Source: CAD feature listing. Evaluate the final solid. Frame: model axes, mm. A direction names the side the tool comes from. Round coordinates to 2 decimals unless told otherwise and drop trailing zeros. Write each loop counter-clockwise with the first axis right and the second up, starting at its lowest first coordinate (ties: lowest second). Pieces come first, ordered by that corner, then holes. Notation, with made-up numbers: (75.25, 22) -> (119.25, 22) arc R14 cw to (119.25, 26) -> close; hole circle Ø6 at (-28.5, -17). An arc over 180 degrees is marked (long way). Put each result on its own line as item: value.
```python
from build123d import *

# Parameters (mm, degrees)
SKETCH2_R           = 0.875
BOSS_EXTRUDE1_DEPTH = 1


with BuildPart() as part:
    # Sketch2 → Boss-Extrude1 (new body)
    with BuildSketch(Plane.XY):
        with BuildLine():
            Line((-5.603408365, 96.42556159), (-5.603408365, 30.425568858))
            ThreePointArc((-5.603408365, 30.425568858), (-4.43183549, 27.597141733), (-1.603408365, 26.425568858))
            Line((-1.603408365, 26.425568858), (41.250894393, 26.425568858))
            ThreePointArc((41.250894393, 26.425568858), (52.580802046, 23.710837368), (61.450097132, 16.156224264))
            Line((61.450097132, 16.156224264), (63.436905361, 13.431841599))
            ThreePointArc((63.436905361, 13.431841599), (64.629324911, 12.347724535), (66.15279536, 11.822165805))
            Line((66.15279536, 11.822165805), (84.159730921, 9.479779923))
            ThreePointArc((84.159730921, 9.479779923), (103.351530482, 5.02611066), (121.297670701, -3.103858071))
            Line((121.297670701, -3.103858071), (122.126093986, -3.582626958))
            ThreePointArc((122.126093986, -3.582626958), (125.162033535, -3.98331921), (127.591695632, -2.119391819))
            Line((127.591695632, -2.119391819), (143.453487011, 25.354036748))
            ThreePointArc((143.453487011, 25.354036748), (143.853088701, 26.318760568), (143.989385396, 27.354036748))
            Line((143.989385396, 27.354036748), (143.989385396, 98.790469349))
            add(Edge.make_bspline(
                [(-5.603408365, 96.42556159), (-5.603408365, 103.460733083), (68.627157279, 109.640132521), (143.989385396, 103.458567417), (143.989385396, 98.790469349)],
                knots=[0, 0, 0, 0, 0.499912399, 1, 1, 1, 1], degree=3))
        make_face()
        with Locations((123.859596668, 0.88165491)):
            Circle(SKETCH2_R, mode=Mode.SUBTRACT)
        with Locations((140.524945013, 32.281066453)):
            Circle(SKETCH2_R, mode=Mode.SUBTRACT)
        with Locations((140.524945013, 55.281066453)):
            Circle(SKETCH2_R, mode=Mode.SUBTRACT)
        with Locations((139.989385396, 97.290469349)):
            Circle(SKETCH2_R, mode=Mode.SUBTRACT)
        with Locations((117.399952063, 99.390469349)):
            Circle(SKETCH2_R, mode=Mode.SUBTRACT)
        with Locations((68.896968427, 102.54989148)):
            Circle(SKETCH2_R, mode=Mode.SUBTRACT)
        with Locations((-1.603408365, 95.42556159)):
            Circle(SKETCH2_R, mode=Mode.SUBTRACT)
        with Locations((-0.871175318, 31.157801905)):
            Circle(SKETCH2_R, mode=Mode.SUBTRACT)
        with Locations((66.6687778, 15.788746464)):
            Circle(SKETCH2_R, mode=Mode.SUBTRACT)
        with BuildLine():
            Line((2.396591635, 90.463437274), (2.396591635, 35.425568858))
            ThreePointArc((2.396591635, 35.425568858), (2.689484854, 34.718462076), (3.396591635, 34.425568858))
            Line((3.396591635, 34.425568858), (39.394762972, 34.425568858))
            ThreePointArc((39.394762972, 34.425568858), (40.101869753, 34.718462076), (40.394762972, 35.425568858))
            Line((40.394762972, 35.425568858), (40.394762972, 38.171054802))
            ThreePointArc((40.394762972, 38.171054802), (40.687656191, 38.878161583), (41.394762972, 39.171054802))
            Line((41.394762972, 39.171054802), (58.395031929, 39.171054802))
            ThreePointArc((58.395031929, 39.171054802), (59.10213871, 39.463948021), (59.395031929, 40.171054802))
            Line((59.395031929, 40.171054802), (59.395031929, 40.549898748))
            ThreePointArc((59.395031929, 40.549898748), (59.687925148, 41.257005529), (60.395031929, 41.549898748))
            Line((60.395031929, 41.549898748), (67.915303846, 41.549898748))
            ThreePointArc((67.915303846, 41.549898748), (68.622863481, 41.256552384), (68.915303025, 40.548617472))
            Line((68.915303025, 40.548617472), (68.889503983, 20.413194101))
            ThreePointArc((68.889503983, 20.413194101), (69.137749853, 19.75246839), (69.760507552, 19.420267661))
            Line((69.760507552, 19.420267661), (106.406539112, 14.653262932))
            ThreePointArc((106.406539112, 14.653262932), (106.598457108, 14.608726239), (106.77791851, 14.527426552))
            Line((106.77791851, 14.527426552), (121.798174914, 5.846802094))
            ThreePointArc((121.798174914, 5.846802094), (122.557159801, 5.746629031), (123.164575325, 6.212610879))
            Line((123.164575325, 6.212610879), (136.560419931, 29.414894346))
            Line((136.560419931, 29.414894346), (136.998243059, 30.153322469))
            ThreePointArc((136.998243059, 30.153322469), (137.105460539, 30.916626107), (136.637925468, 31.529438468))
            Line((136.637925468, 31.529438468), (116.900098761, 42.920620776))
            ThreePointArc((116.900098761, 42.920620776), (116.533969008, 43.286657516), (116.399952063, 43.78673086))
            Line((116.399952063, 43.78673086), (116.399952063, 92.828345033))
            ThreePointArc((116.399952063, 92.828345033), (116.118152375, 93.508669661), (115.437827746, 93.790469349))
            Line((115.437827746, 93.790469349), (98.360317754, 93.790469349))
            ThreePointArc((98.360317754, 93.790469349), (97.679993126, 94.072269037), (97.398193438, 94.752593666))
            Line((97.398193438, 94.752593666), (97.398193438, 95.213192117))
            ThreePointArc((97.398193438, 95.213192117), (97.11639375, 95.893516746), (96.436069121, 96.175316434))
            Line((96.436069121, 96.175316434), (79.359092742, 96.175316434))
            ThreePointArc((79.359092742, 96.175316434), (78.678768113, 96.457116122), (78.396968425, 97.137440751))
            Line((78.396968425, 97.137440751), (78.396968425, 97.587767164))
            ThreePointArc((78.396968425, 97.587767164), (78.115168737, 98.268091793), (77.434844109, 98.54989148))
            Line((77.434844109, 98.54989148), (60.359092745, 98.54989148))
            ThreePointArc((60.359092745, 98.54989148), (59.678768117, 98.268091793), (59.396968429, 97.587767164))
            Line((59.396968429, 97.587767164), (59.396968429, 97.133171852))
            ThreePointArc((59.396968429, 97.133171852), (59.115168741, 96.452847223), (58.434844112, 96.171047535))
            Line((58.434844112, 96.171047535), (41.357156249, 96.171047535))
            ThreePointArc((41.357156249, 96.171047535), (40.676831621, 95.889247847), (40.395031933, 95.208923218))
            Line((40.395031933, 95.208923218), (40.395031933, 92.387685907))
            ThreePointArc((40.395031933, 92.387685907), (40.113232245, 91.707361278), (39.432907616, 91.42556159))
            Line((39.432907616, 91.42556159), (3.358715952, 91.42556159))
            ThreePointArc((3.358715952, 91.42556159), (2.678391323, 91.143761902), (2.396591635, 90.463437274))
        make_face(mode=Mode.SUBTRACT)
    extrude(amount=BOSS_EXTRUDE1_DEPTH)


solid = part.part
```
Q1. Draft query along Y for faces 3 (the flat face through (68, 41, 0)), 4 (the cylindrical face through (-4.463, 27.628, 0.493)), 5 (the flat face through (114.18, 10.25, 0.49)), 6 (the flat face through (87.83, 17.07, 0.49)). Return one class per face: +Y half, -Y half, draft (parallel to the pull), parting line (faces both ways), or undercut.
Ans:
face 3: draft
face 4: -Y half
face 5: undercut
face 6: undercut
Q2. Pin query (flat end, axial travel): pin 1 (0.5 mm diameter, centred on x = 21.5, z = 0.5, fed in from -Y); pin 2 (0.5 mm diameter, centred on x = 52.5, z = 0.5, fed in from +Y). Return the tip coordinate at first contact, or that it passes through.
Ans:
pin 1: stops at y = 26.43
pin 2: stops at y = 106.35
Q3. Cut plane C-C on z = 0.75. Give the number of separate pieces and of enclosed holes in the cut face, and give its area (3 significant figures).
Ans:
separate pieces: 1
enclosed holes: 10
area: 5,290 mm^2
Q4. Material intervals for line 1 (X direction, y = 84, z = 0.8); line 2 (Y direction, x = 117, z = 0.9); line 3 (X direction, y = 95.5, z = 0.35), sorted ascending. Write a range as [from, to].
Ans:
line 1: x = [-5.6, 2.4], [116.4, 143.99]
line 2: y = [-0.76, 8.62], [42.86, 98.61], [100.17, 104.73]
line 3: x = [-5.6, -2.48], [-0.73, 40.44], [97.35, 143.99]
Q5. Reachability of faces 1 (the flat face through (129.77, 17.65, 0.49)), 2 (the cylindrical face through (103.09, 5.114, 0.493)) from +Z, -Z, +X, -X, +Y, -Y: full face, straight path, thin tool, end or side. Return the list, or none.
Ans:
face 1: +Z, -Z
face 2: +Z, -Z, -X, -Y
Q6. Cut plane B-B on y = 23. Output: boundary loops of the cut face in (x, z), and give its area (3 significant figures).
Ans:
outline: (53.88, 0) -> (68.89, 0) -> (68.89, 1) -> (53.88, 1) -> close; (132.86, 0) -> (142.09, 0) -> (142.09, 1) -> (132.86, 1) -> close
area: 24.2 mm^2
Q7. Cut plane A-A on y = 74. Output: boundary loops of the cut face in (x, z), and give its area (3 significant figures).
Ans:
outline: (-5.6, 0) -> (2.4, 0) -> (2.4, 1) -> (-5.6, 1) -> close; (116.4, 0) -> (143.99, 0) -> (143.99, 1) -> (116.4, 1) -> close
area: 35.6 mm^2
Q8. Cut plane D-D on y = 4. Output: boundary loops of the cut face in (x, z), and give its area (3 significant figures).
Ans:
outline: (106.23, 0) -> (131.12, 0) -> (131.12, 1) -> (106.23, 1) -> close
area: 24.9 mm^2
